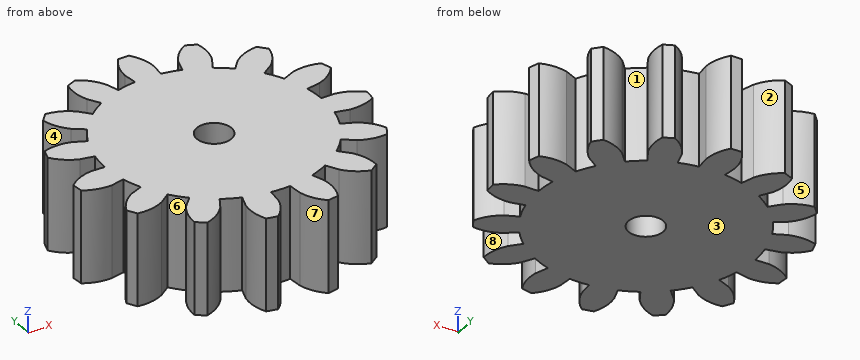
```python
from build123d import *

# Parameters (mm, degrees)
SKETCH2_R           = 9.375
BOSS_EXTRUDE1_DEPTH = 8
BOSS_EXTRUDE2_DEPTH = 8
CIRPATTERN1_COUNT   = 15
SKETCH4_R           = 1.5
CUT_EXTRUDE1_DEPTH  = 8


with BuildPart() as part:
    # Sketch2 → Boss-Extrude1 (new body)
    with BuildSketch(Plane.XY):
        Circle(SKETCH2_R)
    extrude(amount=BOSS_EXTRUDE1_DEPTH)

    # Sketch3 → Boss-Extrude2 (add)
    with BuildSketch(Plane.XY.offset(8)):
        with BuildLine():
            Line((0, 0), (1.26165998, 10.496446927))
            ThreePointArc((1.26165998, 10.496446927), (1.046763133, 11.682170305), (0.471921711, 12.741263277))
            Line((0.471921711, 12.741263277), (-0.471921711, 12.741263277))
            ThreePointArc((-0.471921711, 12.741263277), (-1.046763133, 11.682170305), (-1.26165998, 10.496446927))
            Line((-1.26165998, 10.496446927), (0, 0))
        make_face()
    boss_extrude2 = extrude(amount=-BOSS_EXTRUDE2_DEPTH)

    # CirPattern1: Boss-Extrude2 ×15 about axis
    cirpattern1_axis = Axis((0, 0, 0), (0, 0, 1))
    for i in range(1, CIRPATTERN1_COUNT):
        add(boss_extrude2.rotate(cirpattern1_axis, i * 360 / CIRPATTERN1_COUNT))

    # Sketch4 → Cut-Extrude1 (cut)
    with BuildSketch(Plane.XY.offset(8)):
        Circle(SKETCH4_R)
    extrude(amount=-CUT_EXTRUDE1_DEPTH, mode=Mode.SUBTRACT)


solid = part.part
```
Geometry check sheet. Reference: the model listing, model coordinates, mm. Face numbers are marked on the shaded views. A direction names the side the tool comes from. Coordinates: 2 decimals unless noted, no trailing zeros. Loops run counter-clockwise (first coordinate to the right, second up) from the corner with the lowest first, then second, coordinate; pieces in that order, holes last. Notation, with made-up numbers: (60, -35) - (109, -35) arc R6 ccw to (109, -31) - close; hole circle Ø9 at (43, 89.25). An arc over 180 degrees is marked (long way). One line per item, written item: value. Start each with the question number.
(1) Cross-section at A-A on x = 0. Enter the section's corners in (y, z) (3 decimals).
(2) Material ranges on line 1 (Y direction, x = 0, z = 5) (3 decimals); line 2 (Y direction, x = -10, z = 5.75); line 3 (Y direction, x = -9.5, z = 5), recorded low to high. Write a range as [from, to].
(3) Cross-section at B-B on y = 7.5. Enter the section's corners in (x, z) (3 decimals).
(4) Mould release check, pull along Y, two halves, no side actions. Record for the marked faces 1, 2 and 3: released by +Y, released by -Y, zero draft, split by the parting line, or undercut.
(5) Tool access check on the marked faces 4, 5, 6, 7 and 8. Record the directions out of +Z, -Z, +X, -X, +Y, -Y that give a thin tool (end or side, any length) a straight path to the whole face; none if there is none.
(6) Depth check by flat-ended pin: P1, Ø2.5, axis at x = 0, y = 0, coming from the +Z side; P2, Ø3, axis at y = 8, z = 6, coming from the +X side. Enter the tip coordinate at first touch or a pass-through.
Results below:
1. outline: (-9.375, 0) - (-1.5, 0) - (-1.5, 8) - (-9.375, 8) - close; (1.5, 0) - (12.741, 0) - (12.741, 8) - (1.5, 8) - close
2. line 1: y = [-9.375, -1.5], [1.5, 12.741]
2. line 2: y = [-6.8, -4.34], [-2.28, 0.15], [1.97, 4.54]
2. line 3: y = [-6.73, -4.06], [-2.17, 0.14], [1.87, 4.4], [7.27, 8.49]
3. outline: (-9.595, 0) - (-6.553, 0) - (-6.553, 8) - (-9.595, 8) - close; (-5.625, 0) - (5.625, 0) - (5.625, 8) - (-5.625, 8) - close; (6.553, 0) - (9.595, 0) - (9.595, 8) - (6.553, 8) - close
4. face 1: undercut
4. face 2: released by +Y
4. face 3: zero draft
5. face 4: +Z, -Z, -X
5. face 5: +Z, -Z, +Y
5. face 6: +Z, -Z
5. face 7: +Z, -Z, -Y
5. face 8: +Z, -Z, +X
6. P1: passes through
6. P2: stops at x = 9.78
